Part model, mm, in its own coordinate system. A direction names the side the tool comes from. Give positions to 0.01 mm unless a question says otherwise; leave off trailing zeros. Order: outer loops, then holes, each group sorted by start corner. A loop starts at its lowest first (then second) coordinate and runs counter-clockwise, first axis right, second up.
1. Mould opens along Y. For faces 4 (the flat face through (60, -10, 1)), 5 (the flat face through (-57, -10, 1)), 6 (the flat face through (-58.7, -70, 1)) say: +Y half, -Y half, draft (parallel to the pull), parting line (faces both ways), or undercut.
2. Slice it at B-B on x = 48. List the corners of the cut face in (y, z).
3. Probe line 1 (X direction, y = -37.5, z = 1.8); line 2 (Y direction, x = 12.5, z = 2.1); line 3 (Y direction, x = -16, z = 2.6). List the from-to ranges inside material, lowest first.
4. Slice it at C-C on z = 1.75. Give the number of separate pieces and of enclosed holes in the cut face, and give its area (3 significant figures).
5. Which spindle directions (+Z, -Z, +X, -X, +Y, -Y) get a long thin tool onto all of the face, cutting with end or side? Do faces 1 (the flat face through (41.3, -72, 1)), 2 (the flat face through (-56.1, -37, 1)), 3 (the flat face through (26.3, 3, 1)). Say none if no direction does.
6. Drop flat-ended pins along their axis: pin 1 Ø0.9 at (y, z) = (-70, 1) entering from +X; pin 2 Ø0.9 at (y, z) = (2.5, 1) entering from -X; pin 3 Ø0.8 at (x, z) = (-58, 1) entering from +Y. Give the stop position or say it passes through.
7. Slice it at A-A on y = -43.5. List the corners of the cut face in (x, z), and give its area (3 significant figures).
from build123d import *

# Parameters (mm, degrees)
BOSS_EXTRUDE1_DEPTH = 3
CUT_EXTRUDE1_DEPTH  = 4
CUT_EXTRUDE3_DEPTH  = 4.0000001


with BuildPart() as part:
    # Sketch1 → Boss-Extrude1 (new body)
    with BuildSketch(Plane.XY):
        Polygon((-58.7, -75), (-38.7, -75), (-38.7, -69), (41.3, -69), (41.3, -75), (58.7, -75), (58.7, -65), (61.3, -65), (61.3, -10), (58.7, -10), (58.7, 0), (26.3, 0), (26.3, 6), (-23.7, 6), (-23.7, 0), (-58.7, 0), (-58.7, -10), (-56.1, -10), (-56.1, -65), (-58.7, -65), align=None)
    extrude(amount=BOSS_EXTRUDE1_DEPTH)

    # Sketch2 → Cut-Extrude1 (cut, through all)
    with BuildSketch(Plane(origin=(0, 0, 0), x_dir=(-1, 0, 0), z_dir=(0, 0, -1))):
        with BuildLine():
            add(Edge.make_bspline(
                [(24.433398527, -31.711635794), (12.086875589, -21.375223364), (4.140193098, -35.358229775), (-5.972759652, -39.022471709)],
                knots=[0, 0, 0, 0, 1, 1, 1, 1], degree=3))
            add(Edge.make_bspline(
                [(24.433398527, -31.711635794), (12.266801911, -25.891579846), (4.786651273, -37.542126637), (-5.972759652, -39.022471709)],
                knots=[0, 0, 0, 0, 1, 1, 1, 1], degree=3))
        make_face()
        with BuildLine():
            add(Edge.make_bspline(
                [(19.633876366, -27.309577158), (8.736929361, -24.137857676), (-2.141100893, -40.478091734), (-22.792881591, -41.192187033), (-28.893422578, -33.772468692)],
                knots=[0, 0, 0, 0, 0.516039473, 1, 1, 1, 1], degree=3))
            add(Edge.make_bspline(
                [(19.633876366, -27.309577158), (9.023428577, -20.186786928), (-2.404229512, -35.749210026), (-21.92167278, -39.158153915), (-28.893422578, -33.772468692)],
                knots=[0, 0, 0, 0, 0.521405392, 1, 1, 1, 1], degree=3))
        make_face()
        with BuildLine():
            add(Edge.make_bspline(
                [(8.169819804, -23.626017478), (-3.788465932, -26.918738654), (-12.420801252, -41.286617905), (-27.125100941, -32.24653048)],
                knots=[0, 0, 0, 0, 1, 1, 1, 1], degree=3))
            add(Edge.make_bspline(
                [(8.169819804, -23.626017478), (-4.800169657, -23.753336514), (-12.720211609, -38.015113151), (-27.125100941, -32.24653048)],
                knots=[0, 0, 0, 0, 1, 1, 1, 1], degree=3))
        make_face()
        with BuildLine():
            add(Edge.make_bspline(
                [(-0.374797507, -23.912294014), (-7.802045912, -26.759848505), (-16.403312917, -34.789264508), (-25.125919349, -30.178411592)],
                knots=[0, 0, 0, 0, 1, 1, 1, 1], degree=3))
            add(Edge.make_bspline(
                [(-0.374797507, -23.912294014), (-9.180167192, -24.486819088), (-15.773948384, -32.398766596), (-25.125919349, -30.178411592)],
                knots=[0, 0, 0, 0, 1, 1, 1, 1], degree=3))
        make_face()
    extrude(amount=-CUT_EXTRUDE1_DEPTH, mode=Mode.SUBTRACT)

    # Sketch4 → Cut-Extrude3 (cut, through all)
    with BuildSketch(Plane(origin=(0, 0, 0), x_dir=(-1, 0, 0), z_dir=(0, 0, -1))):
        with BuildLine():
            Line((-41.3, -69), (38.7, -69))
            ThreePointArc((38.7, -69), (-1.3, -59.5572809), (-41.3, -69))
        make_face()
    extrude(amount=-CUT_EXTRUDE3_DEPTH, mode=Mode.SUBTRACT)


solid = part.part
Data:
1. face 4: +Y half
1. face 5: undercut
1. face 6: draft
2. outline: (-75, 0) - (0, 0) - (0, 3) - (-75, 3) - close
3. line 1: x = -56.1 to 0.68, 2.73 to 6.45, 24.52 to 61.3
3. line 2: y = -60.26 to -39.35, -36.3 to -34.31, -31.86 to -29.94, -28.07 to 6
3. line 3: y = -61.25 to -30.2, -27.98 to -26.65, -25.37 to 6
4. separate pieces: 1
4. enclosed holes: 4
4. area: 7,850 mm2
5. face 1: +Z, -Z, -Y
5. face 2: +Z, -Z, -X
5. face 3: +Z, -Z, +X, +Y
6. pin 1: stops at x = 58.7
6. pin 2: stops at x = -23.7
6. pin 3: stops at y = 0
7. outline: (-56.1, 0) - (61.3, 0) - (61.3, 3) - (-56.1, 3) - close
7. area: 352 mm2
